Autodesk Fusion 360 part; units mm, degrees
sketch "Sketch1" plane through (0, 0, 0) normal (0, 1, 0) x (1, 0, 0)
  line L0 (-37, 0) -> (-100, 0)
  line L1 (-100, 0) -> (-100, -10)
  line L2 (-100, -10) -> (-60, -10)
  line L3 (0, -10) -> (0, -5)
  line L4 (-32, -5) -> (-37, 0)
  line L5 (-32, -5) -> (-32, -10)
  line L6 (-40, -85) -> (-50, -85)
  line L7 (-40, -85) -> (-40, -50)
  line L8 (-40, -50) -> (-32, -45)
  line L9 (-50, -75) -> (-60, -75)
  line L10 (-50, -85) -> (-50, -75)
  line L11 (-60, -75) -> (-60, -65)
  line L12 (-60, -65) -> (-57, -65)
  line L13 (-57, -65) -> (-57, -60)
  line L14 (-57, -60) -> (-60, -60)
  line L15 (-32, -5) -> (-32, -15)
  line L16 (-32, -15) -> (-40, -15)
  line L17 (-40, -15) -> (-40, -20)
  line L18 (-40, -20) -> (-32, -20)
  line L19 (-60, -10) -> (-60, -60)
  line L20 (-60, -65) -> (-60, -75)
  line L21 (-32, -5) -> (-32, -15)
  line L22 (-32, -20) -> (-32, -45)
  dimension "d1" = 100
  dimension "d2" = 10
  dimension "d5" = 60
  dimension "d15" = 65
  dimension "d16" = 10
  dimension "d17" = 3
  dimension "d19" = 8
revolve "Revolve1" add sketch "Sketch1" angle 360 about axis through (0, 0, 1.75) along (0, 0, 1) second angle 360
hole "Hole1" at (64.5241, -55.0471, 10) direction (0, 0, -1) diameter 10 depth 10 tip angle 118
pattern_circular "C-Pattern1" count 4 over 360 about axis through (0, 0, 1.75) along (0, 0, 1) of "Hole1"
hole "Hole2" at (-42.4264, -42.4264, 38.7259) direction (0.7071, 0.7071, 0) diameter 6 depth 32 tip angle 118
pattern_circular "C-Pattern2" count 4 over 360 about axis through (0, 0, 1.75) along (0, 0, 1) of "Hole2"
sketch "Sketch2" plane through (0, 0, 0) normal (0, 0, 1) x (1, 0, 0)
  line L0 (0, 0) -> (110, 0)
  line L1 (110, 0) -> (110, -110)
  line L2 (110, -110) -> (0, -110)
  line L3 (0, -110) -> (0, 0)
extrude "Extrude1" cut sketch "Sketch2" along normal blind 110
Design review of the part built by this model. Coordinates are the model's own, in mm. A direction names the side the tool comes from. Give positions to 0.01 mm unless a question says otherwise; leave off trailing zeros. Order: outer loops, then holes, each group sorted by start corner. A loop starts at its lowest first (then second) coordinate and runs counter-clockwise, first axis right, second up. Notation, with made-up numbers: (53.5, 0) -> (84.5, 0) arc R9 ccw to (84.5, 13) -> close; hole circle Ø11 at (3, -7.5). An arc over 180 degrees is marked (long way). Write item = value, one per line. Start each with the question number.
(1) We need section C-C on y = -53.5. Write out the cut boundary in (x, z).
(2) For pin 1 (6 mm diameter, centred on x = -23.5, z = 46.5, fed in from +Y); pin 2 (20.5 mm diameter, centred on y = -51, z = 55, fed in from +X); pin 3 (2 mm diameter, centred on x = 5, z = 60, fed in from -Y), all flat-tipped, find the tip position at first contact; note any pin that passes through.
(3) For faces 1 (the face through (-23.59, 22.08, 4.69)), 2 (the face through (50, 0, 32)), 3 (the face through (-43.803, 41.004, 69.93)), 4 (the face through (-21.87, 23.36, 10.07)), 5 (the face through (-24, 24, 15)), list the 3-axis set-ups (+Z, -Z, +X, -X, +Y, -Y) from which the entire face can be reached by the end or side of a thin tool; tool diameter is ignored.
(4) We need section B-B on z = 24. Write out the cut boundary in (x, y).
(5) Mouldability with a two-part tool opening along Y and no side actions: class faces 6 (the face through (-43, 43, 10)), 7 (the face through (-36.5, 34.17, 79.93)), 8 (the face through (-24, 24, 20)) as +Y half, -Y half, draft (parallel to the pull), parting line (faces both ways), or undercut.
(6) We need section A-A on y = 53. Write out the cut boundary in (x, z).
(7) To check wall thickness, follow line 1 along Z through (x, y) = (-35.5, -84.5); line 2 along Z through (x, y) = (-17.5, -54); line 3 along Y through (x, z) = (-10.5, 8.5). State the ranges of each line that lie inside material, in increasing order.
(8) We need section D-D on x = -77.5. Write out the cut boundary in (y, z).
Numbers:
q1.outline = (-84.49, 0) -> (0, 0) -> (0, 75) -> (-27.16, 75) -> (-27.16, 65) -> (-19.67, 65) -> (-19.67, 60) -> (-27.16, 60) -> (-27.16, 10) -> (-84.49, 10) -> close
q2.pin_1 = 56.39
q2.pin_2 = 0
q2.pin_3 = 39.55
q3.face_1 = -Z
q3.face_2 = +Z, -Z, +X, -Y
q3.face_3 = +Z
q3.face_4 = +Z, -Z
q3.face_5 = none
q4.outline = (0, -60) -> (0, -32) arc R32 cw (long way) to (32, 0) -> (60, 0) arc R60 ccw (long way) to start
q5.face_6 = draft
q5.face_7 = parting line
q5.face_8 = undercut
q6.outline = (-84.8, 0) -> (-69.09, 0) -> (-69.09, 10) -> (-84.8, 10) -> close; (-59.96, 0) -> (84.8, 0) -> (84.8, 10) -> (28.12, 10) -> (28.12, 60) -> (20.98, 60) -> (20.98, 65) -> (28.12, 65) -> (28.12, 75) -> (-28.12, 75) -> (-28.12, 65) -> (-20.98, 65) -> (-20.98, 60) -> (-28.12, 60) -> (-28.12, 10) -> (-59.96, 10) -> close
q7.line_1 = 0 to 10
q7.line_2 = 0 to 75
q7.line_3 = -99.45 to -30.23, 30.23 to 99.45
q8.outline = (-63.2, 0) -> (63.2, 0) -> (63.2, 10) -> (-63.2, 10) -> close
